Read the model definition and answer for the solid it produces. Units are mm, in the model's axes. Give positions to 0.01 mm unless a question says otherwise; leave off trailing zeros. Order: outer loops, then holes, each group sorted by start corner. A loop starts at its lowest first (then second) coordinate and runs counter-clockwise, first axis right, second up. Notation, with made-up numbers: (-1.5, 2) -> (53.5, 2) arc R32 cw to (53.5, 31) -> close; hole circle Ø9 at (-6.75, 72). An arc over 180 degrees is marked (long way). Answer as CSV lines item,"result". Start each with the question number.
1) Straight lines are drawn through the part: L1, parallel to X at y = 0.25, z = 0; L2, parallel to Z at x = 6.5, y = 0.4; L3, parallel to Z at x = 7, y = 0.35. For each, find the intervals that lie inside material, in ascending order. Write a range as from..to.
2) Find section B-B (z = 0). Determine the outline of the cut face in (x, y).
3) Find section A-A (x = 0). Determine the outline of the cut face in (y, z), and give its area (3 significant figures).
4) A flat-ended cylindrical pin translates along its axis: pin 1 Ø1.5 at (x, z) = (-6.5, 7.5) entering from -Y. Find the tip coordinate at first contact, or state that the pin passes through.
5) Find section C-C (y = 0.2). Determine the outline of the cut face in (x, z).
6) The mould has two halves that part along X. Classify faces 1 (the face through (-9.822, 0.246, 4.603)), 2 (the face through (0, 0.5, -8)), 3 (the face through (0.329, 0.246, 7.993)): +X half, -X half, draft (parallel to the pull), parting line (faces both ways), or undercut.
7) Find section D-D (x = 8.5). Determine the outline of the cut face in (y, z).
```python
from build123d import *

# Parameters (mm, degrees)
BOSS_EXTRUDE1_DEPTH = 0.5
FILLET1_R           = 0.1


with BuildPart() as part:
    # Sketch1 → Boss-Extrude1 (new body)
    with BuildSketch(Plane(origin=(0, 0, 0), x_dir=(1, 0, 0), z_dir=(0, 1, 0))):
        with BuildLine():
            Line((7.405833782, -9.18660035), (6.465631312, -9.585692621))
            ThreePointArc((6.465631312, -9.585692621), (5.866379853, -9.095515782), (5.096810535, -9.180006665))
            ThreePointArc((5.096810535, -9.180006665), (-2.64863632, -10.160449087), (-8.929748506, -5.523548825))
            ThreePointArc((-8.929748506, -5.523548825), (-9.83687626, -4.59242065), (-11.052731833, -4.132447099))
            ThreePointArc((-11.052731833, -4.132447099), (3.116261, 11.381077163), (7.405833782, -9.18660035))
        make_face()
        with BuildLine():
            Line((-1.5, 6.5), (1.5, 6.5))
            Line((1.5, 6.5), (1.5, 7.858116823))
            ThreePointArc((1.5, 7.858116823), (0, -8), (-1.5, 7.858116823))
            Line((-1.5, 7.858116823), (-1.5, 6.5))
        make_face(mode=Mode.SUBTRACT)
    extrude(amount=BOSS_EXTRUDE1_DEPTH)

    # Fillet1
    fillet1_edges = [part.edges().sort_by_distance(p)[0] for p in [
        (-1.5, 0.25, -7.858116823),
        (1.5, 0.25, -7.858116823),
    ]]
    fillet(fillet1_edges, radius=FILLET1_R)


solid = part.part
```
Findings below:
1,L1,"-11.8..-8, 8..11.8"
1,L2,"-9.85..-4.66, 4.66..9.57"
1,L3,"-9.5..-3.87, 3.87..9.36"
2,outline,"(-11.8, 0) -> (-8, 0) -> (-8, 0.5) -> (-11.8, 0.5) -> close; (8, 0) -> (11.8, 0) -> (11.8, 0.5) -> (8, 0.5) -> close"
3,outline,"(0, -11.8) -> (0.5, -11.8) -> (0.5, -6.5) -> (0, -6.5) -> close; (0, 8) -> (0.5, 8) -> (0.5, 10.5) -> (0, 10.5) -> close"
3,area,"3.90 mm²"
4,pin 1,"y = 0"
5,outline,"(-11.05, 4.13) arc R11.8 ccw (long way) to (7.41, 9.19) -> (6.47, 9.59) arc R1 cw to (5.1, 9.18) arc R10.5 ccw to (-8.93, 5.52) arc R3 cw to start; hole (-1.62, -7.83) arc R0.1 ccw to (-1.5, -7.74) -> (-1.5, -6.5) -> (1.5, -6.5) -> (1.5, -7.74) arc R0.1 ccw to (1.62, -7.83) arc R8 ccw (long way) to start"
6,face 1,"-X half"
6,face 2,"draft"
6,face 3,"undercut"
7,outline,"(0, -8.18) -> (0.5, -8.18) -> (0.5, 8.18) -> (0, 8.18) -> close"
